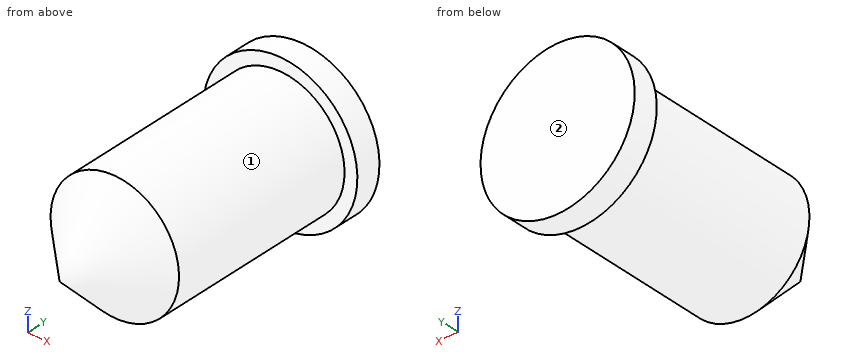
from build123d import *

# Parameters (mm, degrees)
SZKIC1_R                    = 2.5
DODANIE_WYCI_GNI_CIE1_DEPTH = 10
SFAZOWANIE1_SIZE            = 2.5
SZKIC3_R                    = 3
DODANIE_WYCI_GNI_CIE2_DEPTH = 1


with BuildPart() as part:
    # Szkic1 → Dodanie-wyciągnięcie1 (new body)
    with BuildSketch(Plane(origin=(0, 0, 0), x_dir=(1, 0, 0), z_dir=(0, 1, 0))):
        with Locations(Location((0, 0, 0), (0, 0, 270))):
            Circle(SZKIC1_R)
    extrude(amount=DODANIE_WYCI_GNI_CIE1_DEPTH)

    # Sfazowanie1
    sfazowanie1_edges = [part.edges().sort_by_distance(p)[0] for p in [
        (0, 0, -2.5),
    ]]
    chamfer(sfazowanie1_edges, length=SFAZOWANIE1_SIZE)

    # Szkic3 → Dodanie-wyciągnięcie2 (add)
    with BuildSketch(Plane(origin=(0, 10, 0), x_dir=(1, 0, 0), z_dir=(0, 1, 0))):
        with Locations(Location((0, 0, 0), (0, 0, 270))):
            Circle(SZKIC3_R)
    extrude(amount=DODANIE_WYCI_GNI_CIE2_DEPTH)


solid = part.part
Source: CAD feature listing. Evaluate the final solid. Frame: model axes, mm. Face numbers are marked on the shaded views. A direction names the side the tool comes from. Coordinates: 2 decimals unless noted, no trailing zeros. Order: outer loops, then holes, each group sorted by start corner. A loop starts at its lowest first (then second) coordinate and runs counter-clockwise, first axis right, second up. Notation, with made-up numbers: M 38.25,50 L 66.25,50 A15 ccw 66.25,78 Z; hole C 76,74.25 d2. An arc over 180 degrees is marked long. Write each question's results on one line, items separated by ' | '. Start each with the question number.
1. Pin query (flat end, axial travel): pin 1 (1 mm diameter, centred on x = -2, y = 4, fed in from +Z); pin 2 (1.5 mm diameter, centred on y = 9, z = 1.5, fed in from -X); pin 3 (1 mm diameter, centred on x = 1.5, y = 8.5, fed in from +Z). Return the tip coordinate at first contact, or that it passes through.
2. Material intervals for L1, parallel to Y at x = -2.45, z = -1.45; L2, parallel to X at y = 8.75, z = -2; L3, parallel to Y at x = 2.3, z = -0.65, sorted ascending.
3. Section A-A, the plane y = 7.25. Return the cut outline in (x, z), then the cut area to 3 significant figures.
4. Reachability of the marked faces 1 and 2 from +Z, -Z, +X, -X, +Y, -Y: full face, straight path, thin tool, end or side. Return the list, or none.
Solution:
1) pin 1: z = 2 | pin 2: x = -2.38 | pin 3: z = 2.29
2) L1: 10 to 11 | L2: -1.5 to 1.5 | L3: 2.39 to 11
3) outline: C 0,0 d5 | area: 19.6 mm²
4) face 1: -Y | face 2: +Z, -Z, +X, -X, +Y
